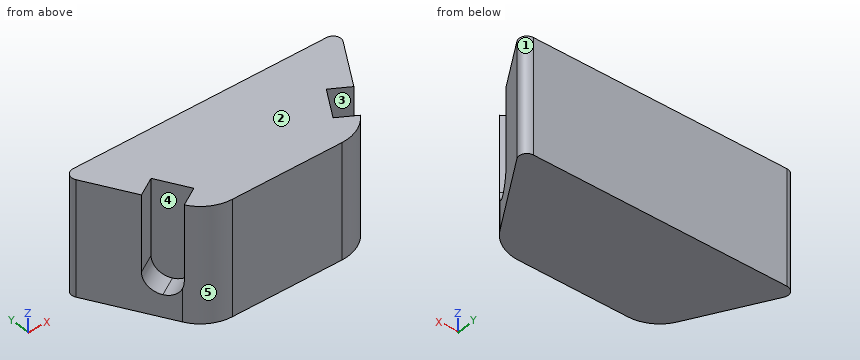
from build123d import *

# Parameters (mm, degrees)
F1_DEPTH = 30
F3_DEPTH = 24.2
F4_R     = 4.49999


# Not quite as in the source:
# - a fillet or chamfer is up to 0.001 mm smaller than in the source, because OpenCascade refuses the exact size


with BuildPart() as f1:
    # F0 (on Top) → F1 (new body)
    with BuildSketch(Plane.XY):
        with BuildLine():
            Line((-13.7223101757, 4.24), (14.2223098243, 4.24))
            ThreePointArc((14.2223098243, 4.24), (19.2223098243, 5.5797459622), (22.8825638622, 9.24))
            Line((22.8825638622, 9.24), (34.2739440306, 28.4706991862))
            ThreePointArc((34.2739440306, 28.4706991862), (34.2907944109, 30.4803025731), (32.5531808711, 31.49))
            Line((32.5531808711, 31.49), (-32.0531791289, 31.49))
            ThreePointArc((-32.0531791289, 31.49), (-33.7907926288, 30.4803026431), (-33.7739423706, 28.4706993249))
            Line((-33.7739423706, 28.4706993249), (-22.3825642135, 9.24))
            ThreePointArc((-22.3825642135, 9.24), (-18.7223101757, 5.5797459622), (-13.7223101757, 4.24))
        make_face()
    extrude(amount=F1_DEPTH)

    # F2 (on face) → F3 (cut)
    with BuildSketch(Plane.XY.offset(30)):
        with BuildLine():
            Line((-26.759759987, 16.6294953398), (-22.3825642135, 9.24))
            ThreePointArc((-22.3825642135, 9.24), (-22.2778836833, 9.0629195529), (-22.1695828196, 8.8880298132))
            Line((-22.1695828196, 8.8880298132), (-17.4408080346, 11.6891376089))
            Line((-17.4408080346, 11.6891376089), (-22.0276610725, 19.4325721963))
            Line((-22.0276610725, 19.4325721963), (-26.759759987, 16.6294953398))
        make_face()
        with BuildLine():
            Line((17.7215177836, 11.3189368702), (22.4312077057, 8.5291335532))
            ThreePointArc((22.4312077057, 8.5291335532), (22.6643714442, 8.879813846), (22.8825638622, 9.24))
            Line((22.8825638622, 9.24), (27.0404701341, 16.2592938501))
            Line((27.0404701341, 16.2592938501), (22.3083714455, 19.0623710879))
            Line((22.3083714455, 19.0623710879), (17.7215177836, 11.3189368702))
        make_face()
    extrude(amount=-F3_DEPTH, mode=Mode.SUBTRACT)

    # F4 (radius 4.5 in the source; OpenCascade refuses exactly that, so slightly less here)
    f4_edges = [f1.edges().sort_by_distance(p)[0] for p in [
        (-24.393711, 18.031034, 5.8),
        (-19.805195, 10.288584, 5.8),
        (24.674421, 17.660832, 5.8),
        (20.076363, 9.924035, 5.8),
    ]]
    fillet(f4_edges, radius=F4_R)


solid = f1.part
Input: part model. Units: mm. Frame: model coordinates. Face numbers are marked on the shaded views. A direction names the side the tool comes from. Give positions to 0.01 mm unless a question says otherwise; leave off trailing zeros. Order: outer loops, then holes, each group sorted by start corner. A loop starts at its lowest first (then second) coordinate and runs counter-clockwise, first axis right, second up. Notation, with made-up numbers: (49.25, -9.75) -> (64.25, -9.75) arc R15 cw to (64.25, -2.75) -> close; hole circle Ø7 at (-6.75, -24). An arc over 180 degrees is marked (long way). Use one line per item in the form item = value.
1) First-contact query: pin 1 Ø1 at (y, z) = (19.5, 12.5) entering from -X; pin 2 Ø1 at (y, z) = (8, 18) entering from -X; pin 3 Ø0.8 at (x, y) = (22, 13.5) entering from +Z. Flat tips, straight axial feed; report the tip coordinate or a pass-through.
Response values:
pin_1 = -28.76
pin_2 = -21.91
pin_3 = 5.88
2) Section A-A, the plane z = 23. Return loops of the section in (x, y).
Response values:
outline = (-33.77, 28.47) -> (-26.76, 16.63) -> (-22.03, 19.43) -> (-17.44, 11.69) -> (-22.17, 8.89) arc R10 ccw to (-13.72, 4.24) -> (14.22, 4.24) arc R10 ccw to (22.43, 8.53) -> (17.72, 11.32) -> (22.31, 19.06) -> (27.04, 16.26) -> (34.27, 28.47) arc R2 ccw to (32.55, 31.49) -> (-32.05, 31.49) arc R2 ccw to start
3) Reachability of the marked faces 4 and 5 from +Z, -Z, +X, -X, +Y, -Y: full face, straight path, thin tool, end or side. Return the list, or none.
Response values:
face_4 = +Z
face_5 = +Z, -Z, -X, -Y
4) Mould query, pull axis X, two halves, no side actions, for the marked faces 1, 2 and 3. Classes: pulls with the +X half, pulls with the -X half, needs draft (parallel to the pull), parting line crosses it, or undercut.
Response values:
face_1 = pulls with the +X half
face_2 = needs draft
face_3 = undercut
5) Line query: probe 1 along X at (y, z) = (17.75, 8.5); probe 2 along X at (y, z) = (17, 15); probe 3 along X at (y, z) = (16.5, 11). Output: solid intervals per line, ascending.
Response values:
probe_1 = -27.42 to -24.13, -21.03 to 21.53, 23.79 to 27.92
probe_2 = -26.98 to -26.13, -20.59 to 21.09, 25.79 to 27.48
probe_3 = -20.29 to 20.79, 26.63 to 27.18
6) Section D-D, the plane z = 9.5. Return loops of the section in (x, y).
Response values:
outline = (-33.77, 28.47) -> (-26.72, 16.57) -> (-21.99, 19.37) -> (-17.48, 11.75) -> (-22.21, 8.95) arc R10 ccw to (-13.72, 4.24) -> (14.22, 4.24) arc R10 ccw to (22.47, 8.59) -> (17.76, 11.38) -> (22.27, 19) -> (27, 16.2) -> (34.27, 28.47) arc R2 ccw to (32.55, 31.49) -> (-32.05, 31.49) arc R2 ccw to start
7) Section B-B, the plane y = 27. Return loops of the section in (x, z), and give its area (3 significant figures).
Response values:
outline = (-32.9, 0) -> (33.4, 0) -> (33.4, 30) -> (-32.9, 30) -> close
area = 1,990 mm^2
8) Section C-C, the plane x = 28. Return loops of the section in (y, z), and give its area (3 significant figures).
Response values:
outline = (17.88, 0) -> (31.49, 0) -> (31.49, 30) -> (17.88, 30) -> close
area = 408 mm^2
